from build123d import *

# Parameters (mm, degrees)
SKETCH1_R                = 29.0703
BOSS_EXTRUDE2_DEPTH      = 4.7625
FILLET1_R                = 3.175
SKETCH2_W                = 14.732
SKETCH2_H                = 10.414
CUT_EXTRUDE2_DEPTH       = 12.7
CIRPATTERN1_COUNT        = 7
SKETCH4_R                = 1.143
CUT_EXTRUDE4_DEPTH       = 9.525
CIRPATTERN2_COUNT        = 7
SKETCH6_R                = 2.159
CUT_EXTRUDE7_DEPTH       = 42.376236281
BOSS_EXTRUDE4_REACH      = 48.843
FILLET2_R                = 0.127
CIRPATTERN5_COUNT        = 7
FILLET2_OF_CIRPATTERN5_R = 0.127
CUT_EXTRUDE9_REACH       = 43.376
SKETCH5_R                = 4.7625
CUT_EXTRUDE8_DEPTH       = 42.376236281
CUT_EXTRUDE8_DEPTH_BACK  = 2.54


with BuildPart() as part:
    # Sketch1 → Boss-Extrude2 (new body)
    with BuildSketch(Plane.XY):
        Circle(SKETCH1_R)
    extrude(amount=-BOSS_EXTRUDE2_DEPTH)

    # Fillet1
    fillet1_edges = [part.edges().sort_by_distance(p)[0] for p in [
        (-29.0703, 0, -4.7625),
    ]]
    fillet(fillet1_edges, radius=FILLET1_R)

    # Sketch2 → Cut-Extrude2 (cut)
    with BuildSketch(Plane.XY):
        with Locations((0, 25.1333)):
            Rectangle(SKETCH2_W, SKETCH2_H)
    cut_extrude2 = extrude(amount=-CUT_EXTRUDE2_DEPTH, mode=Mode.SUBTRACT)

    # CirPattern1: Cut-Extrude2 ×7 about axis
    cirpattern1_axis = Axis((0, 0, 0), (0, 0, 1))
    for i in range(1, CIRPATTERN1_COUNT):
        add(cut_extrude2.rotate(cirpattern1_axis, i * 360 / CIRPATTERN1_COUNT), mode=Mode.SUBTRACT)

    # Sketch4 → Cut-Extrude4 (cut, symmetric)
    with BuildSketch(Plane(origin=(0, 0, 0), x_dir=(0, 0, -1), z_dir=(1, 0, 0))):
        with Locations((0, 25.7683)):
            Circle(SKETCH4_R)
    cut_extrude4 = extrude(amount=CUT_EXTRUDE4_DEPTH, both=True, mode=Mode.SUBTRACT)

    # CirPattern2: Cut-Extrude4 ×7 about axis
    cirpattern2_axis = Axis((0, 0, 0), (0, 0, 1))
    for i in range(1, CIRPATTERN2_COUNT):
        add(cut_extrude4.rotate(cirpattern2_axis, i * 360 / CIRPATTERN2_COUNT), mode=Mode.SUBTRACT)

    # Sketch6 → Cut-Extrude7 (cut, through all)
    with BuildSketch(Plane(origin=(0, 0, -4.7625), x_dir=(-1, 0, 0), z_dir=(0, 0, -1))):
        with Locations((11.1125, 0)):
            Circle(SKETCH6_R)
        with Locations((0, -11.1125)):
            Circle(SKETCH6_R)
        with Locations((-11.1125, 0)):
            Circle(SKETCH6_R)
        with Locations((0, 11.1125)):
            Circle(SKETCH6_R)
    extrude(amount=-CUT_EXTRUDE7_DEPTH, mode=Mode.SUBTRACT)

    # Sketch10 → Boss-Extrude4 (add, up to next)
    with BuildSketch(Plane.ZY.offset(-7.366), mode=Mode.PRIVATE) as boss_extrude4_sk1:
        with BuildLine():
            Line((-4.7625, 19.9263), (0, 19.9263))
            Line((0, 19.9263), (0, 20.0533))
            ThreePointArc((0, 20.0533), (-2.7025038, 20.73265722), (-4.7625, 22.609214887))
            Line((-4.7625, 22.609214887), (-4.7625, 19.9263))
        make_face()
    boss_extrude4_tool1 = extrude(boss_extrude4_sk1.sketch, amount=BOSS_EXTRUDE4_REACH, mode=Mode.PRIVATE) - part.part
    boss_extrude4 = boss_extrude4_tool1.solids().sort_by_distance((7.366, 20.664807, -3.452063))[0]
    add(boss_extrude4)

    # Fillet2
    fillet2_edges = [part.edges().sort_by_distance(p)[0] for p in [
        (0, 22.609214887, -4.7625),
    ]]
    fillet(fillet2_edges, radius=FILLET2_R)

    # CirPattern5: Boss-Extrude4 ×7 about axis
    cirpattern5_axis = Axis((0, 0, 0), (0, 0, 1))
    for i in range(1, CIRPATTERN5_COUNT):
        add(boss_extrude4.rotate(cirpattern5_axis, i * 360 / CIRPATTERN5_COUNT))

    # Fillet2 of CirPattern5
    fillet2_of_cirpattern5_edges = [part.edges().sort_by_distance(p)[0] for p in [
        (-17.676595993, 14.09661491, -4.7625),
        (-22.042354666, -5.031023613, -4.7625),
        (-9.809770694, -20.370198741, -4.7625),
        (9.809770694, -20.370198741, -4.7625),
        (22.042354666, -5.031023613, -4.7625),
        (17.676595993, 14.09661491, -4.7625),
    ]]
    fillet(fillet2_of_cirpattern5_edges, radius=FILLET2_OF_CIRPATTERN5_R)

    # Sketch5 → Cut-Extrude9 (cut, up to next)
    with BuildSketch(Plane.XY, mode=Mode.PRIVATE) as cut_extrude9_sk1:
        Circle(SKETCH5_R)
    cut_extrude9_tool1 = extrude(cut_extrude9_sk1.sketch, amount=-CUT_EXTRUDE9_REACH, mode=Mode.PRIVATE) & part.part
    add(cut_extrude9_tool1.solids().sort_by_distance((0, 0, 0))[0], mode=Mode.SUBTRACT)

    # Sketch7 → Cut-Extrude8 (cut, two sides: drawn at the far end of the back side and taken through both)
    with BuildSketch(Plane(origin=(0, 0, -4.7625), x_dir=(-1, 0, 0), z_dir=(0, 0, -1)).offset(-CUT_EXTRUDE8_DEPTH_BACK)):
        Polygon((15.5575, -2.566321947), (15.5575, 2.566321947), (11.1125, 5.132643893), (6.6675, 2.566321947), (6.6675, -2.566321947), (11.1125, -5.132643893), align=None)
        Polygon((2.566321947, 15.5575), (-2.566321947, 15.5575), (-5.132643893, 11.1125), (-2.566321947, 6.6675), (2.566321947, 6.6675), (5.132643893, 11.1125), align=None)
        Polygon((-2.566321947, -15.5575), (2.566321947, -15.5575), (5.132643893, -11.1125), (2.566321947, -6.6675), (-2.566321947, -6.6675), (-5.132643893, -11.1125), align=None)
        Polygon((-15.5575, 2.566321947), (-15.5575, -2.566321947), (-11.1125, -5.132643893), (-6.6675, -2.566321947), (-6.6675, 2.566321947), (-11.1125, 5.132643893), align=None)
    extrude(amount=CUT_EXTRUDE8_DEPTH + CUT_EXTRUDE8_DEPTH_BACK, mode=Mode.SUBTRACT)


solid = part.part
Work out the finished part from the listing and answer in its coordinate system (mm). A direction names the side the tool comes from. Give positions to 0.01 mm unless a question says otherwise; leave off trailing zeros. Answer as a JSON object with one key per item and string values. Group by question number.
1. Consider line 1 along X through (y, z) = (23, -0.95); line 2 along X through (y, z) = (3, -3); line 3 along X through (y, z) = (-9, -2.35). Determine where each line is inside the solid, lowest interval first. Write a range as [from, to].
2. Section A-A on x = 0 is taken. Count the separate pieces of the cut face and the enclosed holes in it, plus the area to 3 significant figures.
3. A tool of negligible diameter and unlimited length cuts with its end or side. For faces 1 (the flat face through (0, 6.668, -3)), 2 (the cylindrical face through (8.461, 25.743, -1.143)), 3 (the flat face through (14.196, 20.742, -2.348)), from which of +Z, -Z, +X, -X, +Y, -Y can it reach the whole face along a straight path? Write none if from no direction.
4. Flat-ended cylindrical pins translate along their axes: pin 1 Ø1.3 at (y, z) = (-1.5, -3.5) entering from +X; pin 2 Ø2 at (y, z) = (-1, -3) entering from -X; pin 3 Ø1 at (x, z) = (-13.5, -1) entering from +Y; pin 4 Ø2.5 at (x, y) = (11.11, 0) entering from -Z. Find the tip coordinate at first contact, or state that the pin passes through.
5. The mould has two halves that part along X. Classify faces 4 (the flat face through (9, -1, -2.222)), 5 (the cylindrical face through (-28.324, 6.545, -0.783)), 6 (the cylindrical face through (22.679, -18.186, -0.783)): released by +X, released by -X, zero draft, split by the parting line, or undercut.
Result sheet:
{
 "1": {"line 1": "x = [-17.03, -15.43], [-13.8, -7.37], [7.37, 13.8], [15.43, 17.03]", "line 2": "x = [-28.58, -14.81], [-7.42, -3.7], [3.7, 7.42], [14.81, 28.58]", "line 3": "x = [-19.03, -3.91], [3.91, 19.03]"},
 "2": {"separate pieces": "4", "enclosed holes": "0", "area": "126 mm^2"},
 "3": {"face 1": "-Z", "face 2": "+Z", "face 3": "+Z, +X"},
 "4": {"pin 1": "stops at x = 22.07", "pin 2": "stops at x = -22.04", "pin 3": "stops at y = 26", "pin 4": "passes through"},
 "5": {"face 4": "undercut", "face 5": "released by -X", "face 6": "released by +X"}
}
